Design review of the part built by this model. Coordinates are the model's own, in mm. Face numbers are marked on the shaded views. A direction names the side the tool comes from. Round coordinates to 2 decimals unless told otherwise and drop trailing zeros. Write each loop counter-clockwise with the first axis right and the second up, starting at its lowest first coordinate (ties: lowest second). Pieces come first, ordered by that corner, then holes. Notation, with made-up numbers: (-28.5, 72.25) - (-23.5, 72.25) arc R23 cw to (-23.5, 99.25) - close; hole circle Ø3 at (-29.75, 34.25). An arc over 180 degrees is marked (long way). Use one line per item in the form item = value.
```python
from build123d import *

# Parameters (mm, degrees)
BOSS_EXTRUDE1_DEPTH = 14
SKETCH2_R           = 24
SKETCH2_R_2         = 12
BOSS_EXTRUDE2_DEPTH = 18
BOSS_EXTRUDE3_REACH = 178
SKETCH3_W           = 28
SKETCH3_H           = 28
SKETCH5_R           = 12.5
BOSS_EXTRUDE4_DEPTH = 20
CHAMFER1_SIZE       = 2


with BuildPart() as part:
    # Sketch1 → Boss-Extrude1 (new body, symmetric)
    with BuildSketch(Plane.XY):
        with BuildLine():
            Line((0, 32), (18, 32))
            Line((18, 32), (18, 14))
            Line((18, 14), (0, 14))
            ThreePointArc((0, 14), (-14, 0), (0, -14))
            Line((0, -14), (18, -14))
            Line((18, -14), (18, -32))
            Line((18, -32), (0, -32))
            ThreePointArc((0, -32), (-32, 0), (0, 32))
        make_face()
    extrude(amount=BOSS_EXTRUDE1_DEPTH, both=True)

    # Sketch2 → Boss-Extrude2 (add)
    with BuildSketch(Plane(origin=(0, 32, 0), x_dir=(1, 0, 0), z_dir=(0, 1, 0))):
        with Locations((30, 0)):
            Circle(SKETCH2_R)
        with Locations((30, 0)):
            Circle(SKETCH2_R_2, mode=Mode.SUBTRACT)
    boss_extrude2 = extrude(amount=-BOSS_EXTRUDE2_DEPTH)

    # Mirror1: Boss-Extrude2 across plane
    add(boss_extrude2.mirror(Plane.ZX))

    # Sketch3 → Boss-Extrude3 (add, up to next)
    with BuildSketch(Plane(origin=(-122, 0, 0), x_dir=(0, 0, -1), z_dir=(1, 0, 0)), mode=Mode.PRIVATE) as boss_extrude3_sk1:
        Rectangle(SKETCH3_W, SKETCH3_H)
    boss_extrude3_tool1 = extrude(boss_extrude3_sk1.sketch, amount=BOSS_EXTRUDE3_REACH, mode=Mode.PRIVATE) - part.part
    add(boss_extrude3_tool1.solids().sort_by_distance((-122, 0, 0))[0])

    # Sketch4 → Cut-Revolve1 (revolve, cut)
    with BuildSketch(Plane.XY.offset(14)):
        with BuildLine():
            Line((-122, 14), (-122, 7.78))
            Line((-122, 7.78), (-92, 7.78))
            ThreePointArc((-92, 7.78), (-87.601795821, 9.601795821), (-85.78, 14))
            Line((-85.78, 14), (-122, 14))
        make_face()
    cut_revolve1 = revolve(axis=Axis((500000, 14, 14), (-1, 0, 0)), mode=Mode.SUBTRACT)

    # Mirror2: Cut-Revolve1 across plane
    add(cut_revolve1.mirror(Plane.XY), mode=Mode.SUBTRACT)

    # Mirror3: Cut-Revolve1 across plane
    add(cut_revolve1.mirror(Plane.ZX), mode=Mode.SUBTRACT)

    # Mirror3 copy 1 sketch → Mirror3 copy 1 (revolve, cut)
    with BuildSketch(Plane(origin=(0, 0, -14), x_dir=(1, 0, 0), z_dir=(0, 0, -1))):
        with BuildLine():
            Line((-122, 14), (-122, 7.78))
            Line((-122, 7.78), (-92, 7.78))
            ThreePointArc((-92, 7.78), (-87.601795821, 9.601795821), (-85.78, 14))
            Line((-85.78, 14), (-122, 14))
        make_face()
    revolve(axis=Axis((500000, -14, -14), (-1, 0, 0)), mode=Mode.SUBTRACT)

    # Sketch5 → Boss-Extrude4 (add)
    with BuildSketch(Plane.ZY.offset(122)):
        Circle(SKETCH5_R)
    extrude(amount=BOSS_EXTRUDE4_DEPTH)

    # Chamfer1
    chamfer1_edges = [part.edges().sort_by_distance(p)[0] for p in [
        (-142, 0, -12.5),
    ]]
    chamfer(chamfer1_edges, length=CHAMFER1_SIZE)


solid = part.part
```
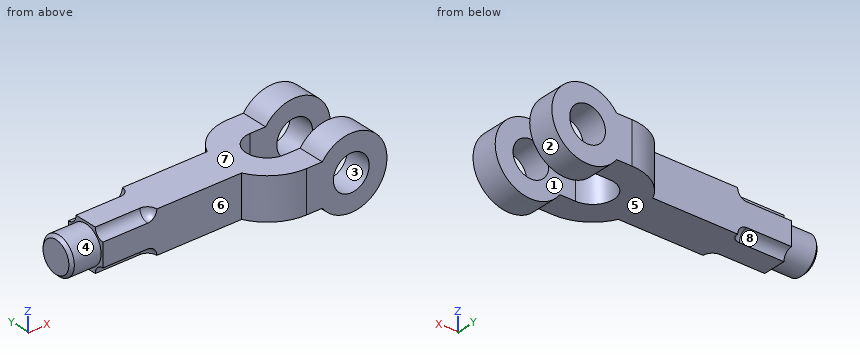
Q1. We need section B-B on z = 0. Write out the cut boundary in (x, y), then the cut area to 3 significant figures.
Calculated:
outline = (-142, -10.5) - (-140, -12.5) - (-122, -12.5) - (-122, -14) - (-28.77, -14) arc R32 ccw to (0, -32) - (18, -32) - (18, -14) - (0, -14) arc R14 cw to (0, 14) - (18, 14) - (18, 32) - (0, 32) arc R32 ccw to (-28.77, 14) - (-122, 14) - (-122, 12.5) - (-140, 12.5) - (-142, 10.5) - close; (42, -32) - (54, -32) - (54, -14) - (42, -14) - close; (42, 14) - (54, 14) - (54, 32) - (42, 32) - close
area = 5,430 mm2
Q2. We need section C-C on x = 30. Write out the cut boundary in (y, z).
Calculated:
outline = (-32, -24) - (-14, -24) - (-14, -12) - (-32, -12) - close; (-32, 12) - (-14, 12) - (-14, 24) - (-32, 24) - close; (14, -24) - (32, -24) - (32, -12) - (14, -12) - close; (14, 12) - (32, 12) - (32, 24) - (14, 24) - close
Q3. We need section D-D on x = -117. Write out the cut boundary in (y, z), then the cut area to 3 significant figures.
Calculated:
outline = (-14, -7.78) arc R6.22 cw to (-7.78, -14) - (7.78, -14) arc R6.22 cw to (14, -7.78) - (14, 7.78) arc R6.22 cw to (7.78, 14) - (-7.78, 14) arc R6.22 cw to (-14, 7.78) - close
area = 662 mm2
Q4. Machinability: for the marked faces 4, 5, 6, 7 and 8, which of the approach directions +Z, -Z, +X, -X, +Y, -Y give a long, thin tool a straight path to every point of the face, cutting with its end or side? Answer none if there is none.
Calculated:
face_4 = -X
face_5 = -Z, -X, +Y, -Y
face_6 = +Z, -Z, -X, -Y
face_7 = +Z, -X, +Y, -Y
face_8 = -Z, -X, +Y
Q5. Draft analysis for pull direction X (two halves, no side actions). For the marked faces 1, 2 and 3, state which applies: released by +X, released by -X, zero draft, split by the parting line, or undercut.
Calculated:
face_1 = zero draft
face_2 = split by the parting line
face_3 = undercut
Q6. To check wall thickness, follow line 1 along Z through (x, y) = (30, 22.75); line 2 along Y through (x, z) = (1, 12.5); line 3 along Z through (x, y) = (-4, 17). State the ranges of each line that lie inside material, in increasing order. Write a range as from..to.
Calculated:
line_1 = -24..-12, 12..24
line_2 = -32..-14, 14..32
line_3 = -14..14
Q7. We need section A-A on x = 6. Write out the cut boundary in (y, z), then the cut area to 3 significant figures.
Calculated:
outline = (-32, -14) - (-14, -14) - (-14, 14) - (-32, 14) - close; (14, -14) - (32, -14) - (32, 14) - (14, 14) - close
area = 1,010 mm2
Q8. For P1, Ø2, axis at x = -108, z = -12.5, coming from the -Y side; P2, Ø2, axis at x = -114.5, z = 11.5, coming from the +Y side; P3, Ø3, axis at x = -51.5, z = 0.5, coming from the +Y side, all flat-tipped, find the tip position at first contact; note any pin that passes through.
Calculated:
P1 = -8.3
P2 = 8.86
P3 = 14
